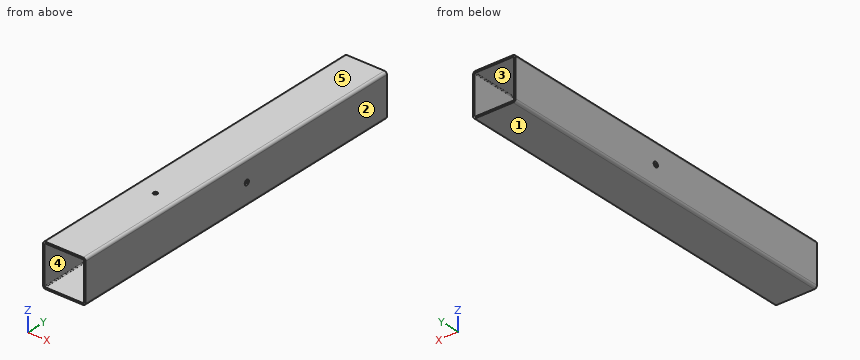
from build123d import *

# Parameters (mm, degrees)
F0_W     = 50
F0_H     = 50
F0_W_2   = 46
F0_H_2   = 46
F1_DEPTH = 430
F2_R     = 1
F3_R     = 3
F4_R     = 2.5
F5_DEPTH = 5
F6_R     = 3
F7_DEPTH = 50.001


with BuildPart() as f1:
    # F0 (on Front) → F1 (new body)
    with BuildSketch(Plane.XZ):
        Rectangle(F0_W, F0_H)
        Rectangle(F0_W_2, F0_H_2, mode=Mode.SUBTRACT)
    extrude(amount=F1_DEPTH)

    # F2
    f2_edges = [f1.edges().sort_by_distance(p)[0] for p in [
        (-23, -215, 23),
        (23, -215, 23),
        (23, -215, -23),
        (-23, -215, -23),
    ]]
    fillet(f2_edges, radius=F2_R)

    # F3
    f3_edges = [f1.edges().sort_by_distance(p)[0] for p in [
        (25, -215, 25),
        (-25, -215, 25),
        (25, -215, -25),
        (-25, -215, -25),
    ]]
    fillet(f3_edges, radius=F3_R)

    # F4 (on face) → F5 (cut)
    with BuildSketch(Plane.XY.offset(25)):
        with Locations((0, -300)):
            Circle(F4_R)
    extrude(amount=-F5_DEPTH, mode=Mode.SUBTRACT)

    # F6 (on face) → F7 (cut, through all)
    with BuildSketch(Plane.YZ.offset(25)):
        with Locations((-200, 0)):
            Circle(F6_R)
    extrude(amount=-F7_DEPTH, mode=Mode.SUBTRACT)


solid = f1.part
Can you work these out from the model? Positions are in its coordinate system, mm. Face numbers are marked on the shaded views. A direction names the side the tool comes from. Give positions to 0.01 mm unless a question says otherwise; leave off trailing zeros. Write each loop counter-clockwise with the first axis right and the second up, starting at its lowest first coordinate (ties: lowest second). Pieces come first, ordered by that corner, then holes. Notation, with made-up numbers: M 44,-3 L 65,-3 A10 cw 65,14 Z; hole C 76,17.25 d11. An arc over 180 degrees is marked long. Answer in a Markdown table with one row per item. Add a question column.
Item 1: For pin 1 Ø3 at (x, y) = (0, -300) entering from +Z, with a flat end and sliding along its axis, tell me the tip position at first contact or that it passes through.
Item 2: Imagine slicing it at A-A, the plane z = 13. Write out the boundary of the cut face in (x, y), plus the area to 3 significant figures.
Item 3: Imagine slicing it at C-C, the plane y = -264.5. Write out the boundary of the cut face in (x, z), plus the area to 3 significant figures.
Item 4: Please list where these lines run through material, in increasing order: L1, parallel to Z at x = 12, y = -411; L2, parallel to X at y = -300, z = 23.85.
Item 5: On a 3-axis mill with a long thin cutter (end or side, diameter ignored), from which of +Z, -Z, +X, -X, +Y, -Y can I reach the whole of each face in a straight line? I mean the marked faces 4 and 5. Say none if no direction works.
Item 6: Imagine slicing it at B-B, the plane x = 12. Write out the boundary of the cut face in (y, z).
Item 7: We'd pull the mould along X, two halves only. Please class the marked faces 1, 2 and 3: released by +X, released by -X, zero draft, split by the parting line, or undercut.
Evaluation:
| question | item | result |
|---|---|---|
| 1 | pin 1 | stops at z = -23 |
| 2 | outline | M -25,-430 L -23,-430 L -23,0 L -25,0 Z; M 23,-430 L 25,-430 L 25,0 L 23,0 Z |
| 2 | area | 1,720 mm² |
| 3 | outline | M -25,-22 A3 ccw -22,-25 L 22,-25 A3 ccw 25,-22 L 25,22 A3 ccw 22,25 L -22,25 A3 ccw -25,22 Z; hole M -23,-22 A1 ccw -22,-23 L 22,-23 A1 ccw 23,-22 L 23,22 A1 ccw 22,23 L -22,23 A1 ccw -23,22 Z |
| 3 | area | 377 mm² |
| 4 | L1 | z = -25 to -23, 23 to 25 |
| 4 | L2 | x = -24.36 to -2.5, 2.5 to 24.36 |
| 5 | face 4 | +Y, -Y |
| 5 | face 5 | +Z, +X, -X, +Y, -Y |
| 6 | outline | M -430,-25 L 0,-25 L 0,-23 L -430,-23 Z; M -430,23 L 0,23 L 0,25 L -430,25 Z |
| 7 | face 1 | zero draft |
| 7 | face 2 | released by +X |
| 7 | face 3 | undercut |
